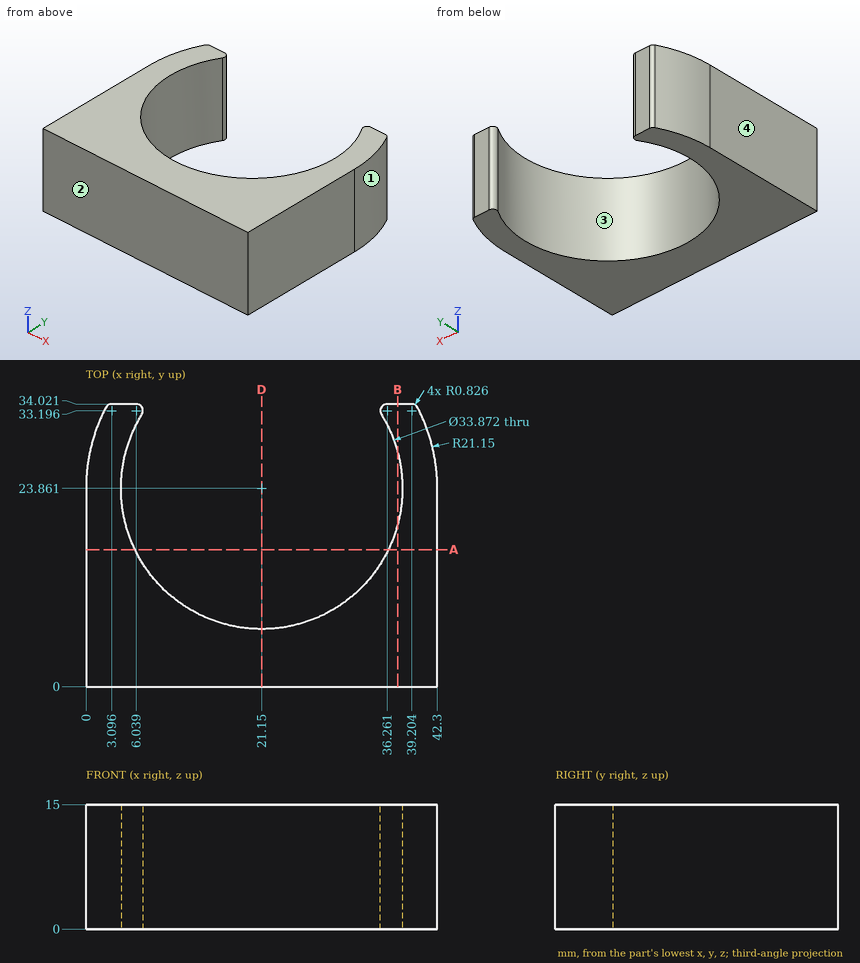
Verification items for this drawing (mm, ordinates from the low corner). Give positions to 0.01 mm unless a question says otherwise; leave off trailing zeros. Write each loop counter-clockwise with the first axis right and the second up, starting at its lowest first coordinate (ties: lowest second). Pieces come first, ordered by that corner, then holes.
1) Section check D-D, the plane x = 21.15. Record the boundary of the cut face in (y, z) (1 decimal).
2) Gauge pin test, flat ends, axial feed: pin 1 (2 mm diameter, centred on x = 12.5, z = 13, fed in from +Y); pin 2 (3 mm diameter, centred on y = 26.5, z = 8.5, fed in from -X); pin 3 (1.5 mm diameter, centred on y = 29.5, z = 10, fed in from -X); pin 4 (10 mm diameter, centred on x = 25.5, y = 14, fed in from -Z). Record the tip position at first contact, or that the pin passes through.
3) Material ranges on L1, parallel to X at y = 9, z = 12.5 (1 decimal); L2, parallel to X at y = 18, z = 11; L3, parallel to Y at x = 21.15, z = 4.75 (1 decimal), recorded low to high.
4) Release check for a two-part mould opening along X. For the marked faces 1, 2, 3 and 4 record: pulls with the +X half, pulls with the -X half, needs draft (parallel to the pull), parting line crosses it, or undercut.
5) Section check B-B, the plane x = 37.5. Record the boundary of the cut face in (y, z), and give its area (3 significant figures).
6) Section check A-A, the plane y = 16.5. Record the boundary of the cut face in (x, z), and give its area (3 significant figures).
Computed:
1. outline: (0, 0) - (6.9, 0) - (6.9, 15) - (0, 15) - close
2. pin 1: stops at y = 9.94
2. pin 2: stops at x = 0.03
2. pin 3: stops at x = 0.57
2. pin 4: passes through
3. L1: x = 0 to 13, 29.3 to 42.3
3. L2: x = 0 to 5.26, 37.04 to 42.3
3. L3: y = 0 to 6.9
4. face 1: pulls with the +X half
4. face 2: needs draft
4. face 3: undercut
4. face 4: pulls with the -X half
5. outline: (0, 0) - (19.44, 0) - (19.44, 15) - (0, 15) - close; (28.28, 0) - (34.02, 0) - (34.02, 15) - (28.28, 15) - close
5. area: 378 mm2
6. outline: (0, 0) - (5.9, 0) - (5.9, 15) - (0, 15) - close; (36.4, 0) - (42.3, 0) - (42.3, 15) - (36.4, 15) - close
6. area: 177 mm2
